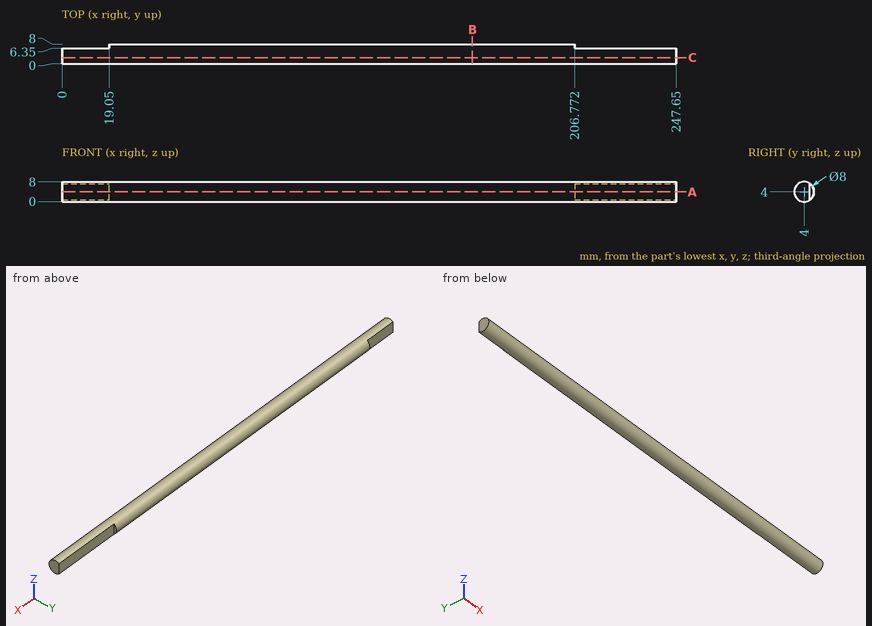
Study the drawing (mm; zero at the part's minimum x, y, z) and answer. Give positions to 0.01 mm unless a question says otherwise; leave off trailing zeros. Order: outer loops, then holes, each group sorted by start corner. A loop starts at its lowest first (then second) coordinate and runs counter-clockwise, first axis right, second up.
1. Each of these flat-tipped pins is pushed along its axis until it touches: P1, Ø4, axis at x = 146, y = 1.5, coming from the -Z side; P2, Ø3, axis at x = 214, z = 6.5, coming from the -Y side; P3, Ø0.8, axis at y = 7, z = 5, coming from the -X side. Where does it stop, or does it pass through?
Result sheet:
P1: stops at z = 0.03
P2: stops at y = 0.13
P3: stops at x = 19.05
2. Section A-A, the plane z = 4 is taken. Determine the outline of the cut face in (x, y), and give its area (3 significant figures).
Result sheet:
outline: (0, 0) - (247.65, 0) - (247.65, 6.35) - (206.77, 6.35) - (206.77, 8) - (19.05, 8) - (19.05, 6.35) - (0, 6.35) - close
area: 1,880 mm2
3. Section C-C, the plane y = 2.5 is taken. Determine the outline of the cut face in (x, z).
Result sheet:
outline: (0, 0.29) - (247.65, 0.29) - (247.65, 7.71) - (0, 7.71) - close
4. Section B-B, the plane x = 165.5 is taken. Determine the outline of the cut face in (y, z), and give its area (3 significant figures).
Result sheet:
outline: circle Ø8 at (4, 4)
area: 50.3 mm2
5. Straight lines are drawn through the part: L1, parallel to X at y = 7, z = 2.25; L2, parallel to Y at x = 130, z = 3.5; L3, parallel to Y at x = 135, z = 6.5. For each, find the intervals that lie inside material, in ascending order.
Result sheet:
L1: x = 19.05 to 206.77
L2: y = 0.03 to 7.97
L3: y = 0.88 to 7.12
